Verification items for this drawing (mm, ordinates from the low corner). Coordinates: 2 decimals unless noted, no trailing zeros. Loops run counter-clockwise (first coordinate to the right, second up) from the corner with the lowest first, then second, coordinate; pieces in that order, holes last. Notation, with made-up numbers: (81, 58.25) -> (98, 58.25) arc R35 cw to (98, 90.25) -> close; hole circle Ø5 at (-12.75, -37). An arc over 180 degrees is marked (long way). Write item = value, one per line.
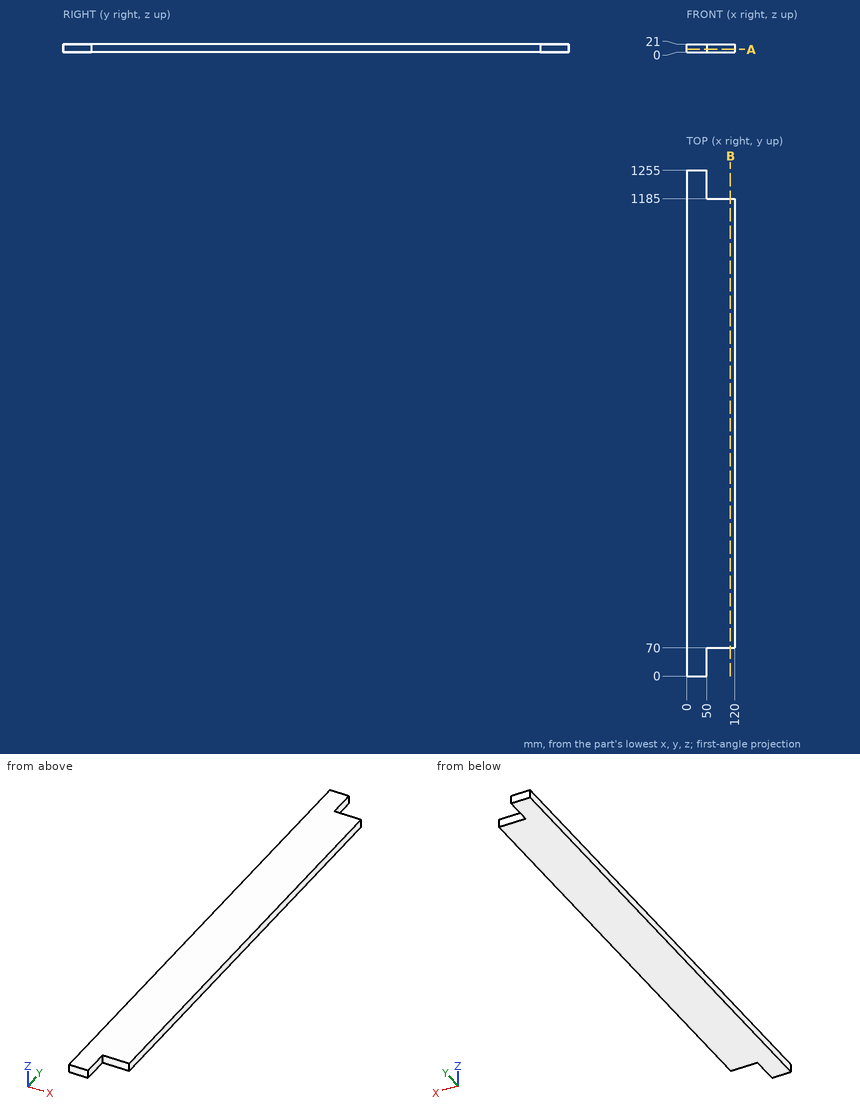
1) Material ranges on line 1 (Y direction, x = 104.5, z = 7.25), recorded low to high.
Ans:
line_1 = 70 to 1185
2) Sectioned sample at B-B, the plane x = 108.5. Record the cut outline in (y, z), plus the area to 3 significant figures.
Ans:
outline = (70, 0) -> (1185, 0) -> (1185, 21) -> (70, 21) -> close
area = 23,400 mm2
3) Sectioned sample at A-A, the plane z = 7.75. Record the cut outline in (x, y).
Ans:
outline = (0, 0) -> (50, 0) -> (50, 70) -> (120, 70) -> (120, 1185) -> (50, 1185) -> (50, 1255) -> (0, 1255) -> close
4) Depth check by flat-ended pin: pin 1 Ø10.5 at (x, z) = (101.5, 6.5) entering from -Y; pin 2 Ø6.5 at (y, z) = (1205.5, 8.5) entering from +X. Enter the tip coordinate at first touch or a pass-through.
Ans:
pin_1 = 70
pin_2 = 50
